Check sheet for the modelled part. Datum: model origin and axes. Units: mm. A direction names the side the tool comes from. Coordinates: 2 decimals unless noted, no trailing zeros. Order: outer loops, then holes, each group sorted by start corner. A loop starts at its lowest first (then second) coordinate and runs counter-clockwise, first axis right, second up.
from build123d import *

# Parameters (mm, degrees)
SKETCH1_W           = 122
SKETCH1_H           = 8
SKETCH1_R           = 1.5
BOSS_EXTRUDE1_DEPTH = 2
SKETCH1_5_R         = 1.5
BOSS_EXTRUDE3_DEPTH = 8


with BuildPart() as part:
    # Sketch1 → Boss-Extrude1 (new body)
    # profile 1 of 4: a face of its own
    with BuildSketch(Plane(origin=(0, 0, 0), x_dir=(1, 0, 0), z_dir=(0, 1, 0))):
        with Locations((0, -35.37)):
            Rectangle(SKETCH1_W, SKETCH1_H)
    # profile 2 of 4: a face of its own
    with BuildSketch(Plane(origin=(0, 0, 0), x_dir=(1, 0, 0), z_dir=(0, 1, 0))):
        Polygon((61, -31.37), (61, -39.37), (66.42, -39.37), (66.42, 39.37), (61, 39.37), (61, 36.37), align=None)
        with Locations(Location((63.75, -36.7, 0), (0, 0, 270))):
            Circle(SKETCH1_R, mode=Mode.SUBTRACT)
        with Locations(Location((63.75, 36.7, 0), (0, 0, 270))):
            Circle(SKETCH1_R, mode=Mode.SUBTRACT)
    # profile 3 of 4: a face of its own
    with BuildSketch(Plane(origin=(0, 0, 0), x_dir=(1, 0, 0), z_dir=(0, 1, 0))):
        Polygon((-61, 39.37), (-61, 36.37), (61, 36.37), (61, 39.37), (-58.92, 39.37), align=None)
    # profile 4 of 4: a face of its own
    with BuildSketch(Plane(origin=(0, 0, 0), x_dir=(1, 0, 0), z_dir=(0, 1, 0))):
        Polygon((-66.42, 31.87), (-66.42, -39.37), (-61, -39.37), (-61, -31.37), (-61, 36.37), (-61, 39.37), (-66.42, 39.37), align=None)
        with Locations(Location((-63.75, -36.7, 0), (0, 0, 270))):
            Circle(SKETCH1_R, mode=Mode.SUBTRACT)
        with Locations(Location((-63.75, 36.7, 0), (0, 0, 270))):
            Circle(SKETCH1_R, mode=Mode.SUBTRACT)
    extrude(amount=BOSS_EXTRUDE1_DEPTH)

    # Sketch1_5 → Boss-Extrude3 (add)
    # profile 1 of 2: a face of its own
    with BuildSketch(Plane(origin=(0, 0, 0), x_dir=(1, 0, 0), z_dir=(0, 1, 0))):
        Polygon((-66.42, 31.87), (-66.42, -39.37), (-61, -39.37), (-61, -31.37), (-61, 36.37), (-61, 39.37), (-66.42, 39.37), align=None)
        with Locations(Location((-63.75, -36.7, 0), (0, 0, 270))):
            Circle(SKETCH1_5_R, mode=Mode.SUBTRACT)
        with Locations(Location((-63.75, 36.7, 0), (0, 0, 270))):
            Circle(SKETCH1_5_R, mode=Mode.SUBTRACT)
    # profile 2 of 2: a face of its own
    with BuildSketch(Plane(origin=(0, 0, 0), x_dir=(1, 0, 0), z_dir=(0, 1, 0))):
        Polygon((61, -31.37), (61, -39.37), (66.42, -39.37), (66.42, 39.37), (61, 39.37), (61, 36.37), align=None)
        with Locations(Location((63.75, -36.7, 0), (0, 0, 270))):
            Circle(SKETCH1_5_R, mode=Mode.SUBTRACT)
        with Locations(Location((63.75, 36.7, 0), (0, 0, 270))):
            Circle(SKETCH1_5_R, mode=Mode.SUBTRACT)
    extrude(amount=BOSS_EXTRUDE3_DEPTH)


solid = part.part
(1) Cross-section at B-B (z = 36.7). Enter the section's corners in (x, y), and give its area (3 significant figures).
Filled in:
outline: (-66.42, 0) - (-65.25, 0) - (-65.25, 8) - (-66.42, 8) - close; (-62.25, 0) - (62.25, 0) - (62.25, 8) - (61, 8) - (61, 2) - (-61, 2) - (-61, 8) - (-62.25, 8) - close; (65.25, 0) - (66.42, 0) - (66.42, 8) - (65.25, 8) - close
area: 283 mm2
(2) Cross-section at D-D (z = -28). Enter the section's corners in (x, y), and give its area (3 significant figures).
Filled in:
outline: (-66.42, 0) - (-61, 0) - (-61, 8) - (-66.42, 8) - close; (61, 0) - (66.42, 0) - (66.42, 8) - (61, 8) - close
area: 86.7 mm2
(3) Cross-section at C-C (x = -17). Enter the section's corners in (y, z), and give its area (3 significant figures).
Filled in:
outline: (0, -39.37) - (2, -39.37) - (2, -36.37) - (0, -36.37) - close; (0, 31.37) - (2, 31.37) - (2, 39.37) - (0, 39.37) - close
area: 22.0 mm2
(4) Tool access check on faces 5 (the flat face through (-66.42, 4, -1)), 6 (the flat face through (-1, 2, 35)). Record the directions out of +Z, -Z, +X, -X, +Y, -Y that give a thin tool (end or side, any length) a straight path to the whole face; none if there is none.
Filled in:
face 5: +Z, -Z, -X, +Y, -Y
face 6: +Z, -Z, +Y
(5) Cross-section at A-A (y = 4.25). Enter the section's corners in (x, z), and give its area (3 significant figures).
Filled in:
outline: (-66.42, -39.37) - (-61, -39.37) - (-61, 39.37) - (-66.42, 39.37) - close; (61, -39.37) - (66.42, -39.37) - (66.42, 39.37) - (61, 39.37) - close; hole circle Ø3 at (-63.75, -36.7); hole circle Ø3 at (-63.75, 36.7); hole circle Ø3 at (63.75, -36.7); hole circle Ø3 at (63.75, 36.7)
area: 825 mm2
(6) Go/stop test with flat-tipped pins: P1, Ø2.5, axis at x = -63.75, z = 36.7, coming from the -Y side; P2, Ø0.9, axis at x = 30.5, z = -38, coming from the +Y side. Record where each tip stops, or that it passes through.
Filled in:
P1: passes through
P2: stops at y = 2
(7) Release check for a two-part mould opening along Z. For faces 1 (the flat face through (64, 8, -1)), 2 (the flat face through (-61, 4, 1)), 3 (the cylindrical face through (-63.3, 3.94, -35.27)), 4 (the flat face through (0.3, 1.6, -39.37)) record: +Z half, -Z half, draft (parallel to the pull), parting line (faces both ways), or undercut.
Filled in:
face 1: draft
face 2: undercut
face 3: undercut
face 4: -Z half
(8) Thickness scan on probe 1 along X at (y, z) = (2.5, -36.7); probe 2 along X at (y, z) = (3, -29); probe 3 along X at (y, z) = (5, -35.5). Record the ranges inside material, lowest first.
Filled in:
probe 1: x = -66.42 to -65.25, -62.25 to -61, 61 to 62.25, 65.25 to 66.42
probe 2: x = -66.42 to -61, 61 to 66.42
probe 3: x = -66.42 to -64.65, -62.85 to -61, 61 to 62.85, 64.65 to 66.42
